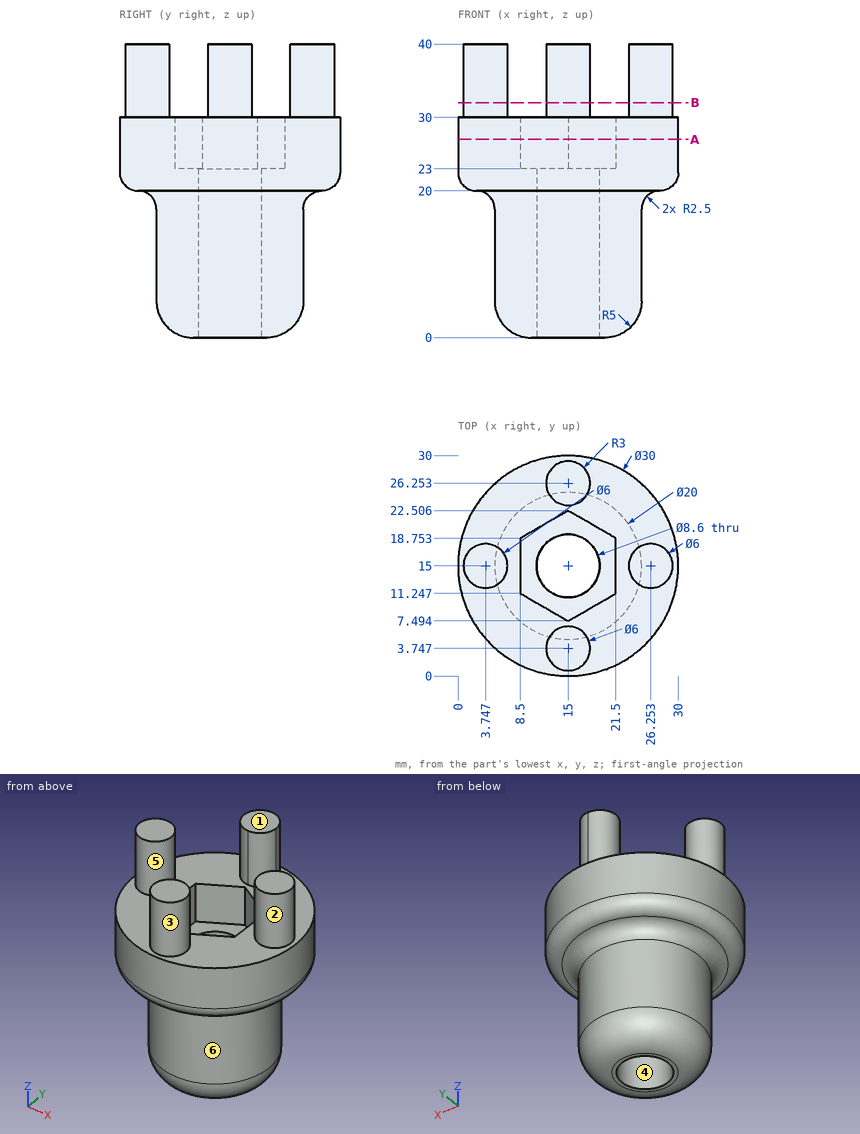
Can you work these out from the drawing? Everything is in mm from the part's minimum corner. A direction names the side the tool comes from. Give positions to 0.01 mm unless a question says otherwise; leave off trailing zeros. Order: outer loops, then holes, each group sorted by start corner. A loop starts at its lowest first (then second) coordinate and runs counter-clockwise, first axis right, second up.
1. I need wall thicknesses on L1, parallel to Y at x = 15, z = 12.5; L2, parallel to X at y = 13.5, z = 27.5 (1 decimal); L3, parallel to Z at x = 2.75, y = 17. Which ranges of each line are inside material? Lowest first, please.
2. Suppose I cut it at B-B (z = 32). List the corners of the cut face in (x, y) for me.
3. Suppose I cut it at A-A (z = 27). List the corners of the cut face in (x, y) for me (1 decimal).
4. For the marked faces 4, 5 and 6, which set-ups out of +Z, -Z, +X, -X, +Y, -Y let a thin tool reach every point of the face, with its end or its side?
5. Will these pins go through, and if not, where does the flat tip stop? P1, Ø10, axis at x = 3, z = 9.5, coming from the -Y side; P2, Ø1.5, axis at y = 4.5, z = 22.5, coming from the -X side; P3, Ø3, axis at x = 11, y = 9.5, coming from the -Z side.
6. We'd pull the mould along X, two halves only. Please class the marked faces 1, 2 and 3: pulls with the +X half, pulls with the -X half, needs draft (parallel to the pull), parting line crosses it, or undercut.
Solved:
1. L1: y = 5 to 10.7, 19.3 to 25
1. L2: x = 0.1 to 8.5, 21.5 to 29.9
1. L3: z = 20 to 40
2. outline: circle Ø6 at (3.75, 15); circle Ø6 at (15, 3.75); circle Ø6 at (15, 26.25); circle Ø6 at (26.25, 15)
3. outline: circle Ø30 at (15, 15); hole (8.5, 11.2) - (15, 7.5) - (21.5, 11.2) - (21.5, 18.8) - (15, 22.5) - (8.5, 18.8) - close
4. face 4: +Z, -Z
4. face 5: +Z
4. face 6: -Z
5. P1: stops at y = 7.86
5. P2: stops at x = 3.6
5. P3: stops at z = 0.01
6. face 1: needs draft
6. face 2: undercut
6. face 3: parting line crosses it
